CAD build for the part. Positions are in the model's coordinates, mm. A direction names the side the tool comes from. Coordinates: 2 decimals unless noted, no trailing zeros. Write each loop counter-clockwise with the first axis right and the second up, starting at its lowest first coordinate (ties: lowest second). Pieces come first, ordered by that corner, then holes. Notation, with made-up numbers: (-34.75, -34.5) -> (-11.75, -34.5) arc R31 cw to (-11.75, -0.5) -> close; hole circle Ø5 at (50.5, -31). An arc over 180 degrees is marked (long way). Answer as CSV lines item,"result".
Autodesk Inventor part; units mm, degrees
ref_plane "Work Plane1" through (0, 0, -3.5) normal (0, 0, 1) x (1, 0, 0)
ref_plane "YZ Plane" through (0, 0, 0) normal (1, 0, 0) x (0, 1, 0)
ref_plane "XZ Plane" through (0, 0, 0) normal (0, 1, 0) x (-1, 0, 0)
sketch "Sketch1" plane through (0, 0, 0) normal (0, 0, 1) x (1, 0, 0)
  line L0 (-8.12, 0) -> (8.12, 0)
  line L1 (0, -19.7) -> (0, 10.05)
  circle A0 centre (0, 0) radius 5.8
  line L2 (-5.8, -15.45) -> (5.8, -15.45)
  line L3 (5.8, -15.45) -> (5.8, 5.8)
  line L4 (5.8, 5.8) -> (-5.8, 5.8)
  line L5 (-5.8, 5.8) -> (-5.8, -15.45)
  line L6 (-5.8, -15.45) -> (5.8, 5.8) construction
  line L7 (5.8, -15.45) -> (-5.8, 5.8) construction
  circle A1 centre (0, -5.95) radius 3
  point P0 (0, -4.825)
  point P1 (0, -8.95)
  dimension "d4" = 6
  dimension "d0" = 21.25
  dimension "d1" = 11.6
  dimension "d5" = 6.5
extrude "Extrusion1" add sketch "Sketch1" against normal blind 20.2
extrude "Extrusion2" add sketch "Sketch1" along normal blind 3.35 contours A0 L1 L0 | L0 L1 A1 A0 | L1 A0 L0 | L0 A0 A1 L1 | A1 L1 A0 | A0 L1 A1 | A1 A0 L1 | A0 A1 L1
sketch "Sketch2" plane through (0, 0, 3.35) normal (0, 0, 1) x (1, 0, 0)
  arc A0 (2.8604, -5.0456) -> (-2.8604, -5.0456) centre (0, 0) ccw
  arc A1 (-2.8604, -5.0456) -> (2.8604, -5.0456) centre (0, -5.95) ccw
  circle A2 centre (0, -5.95) radius 1
  circle A3 centre (0, 0) radius 2.85
  circle A4 centre (0, 0) radius 1.9
  circle A5 centre (0, 0) radius 1.875
  circle A6 centre (0, 0) radius 0.675
  dimension "d9" = 5.7
  dimension "d10" = 2
  dimension "d11" = 3.8
  dimension "d14" = 3.75
  dimension "d17" = 1.35
extrude "Extrusion3" add sketch "Sketch2" along normal blind 0.6 contours A2 | A3
extrude "Extrusion4" add sketch "Sketch2" along normal blind 2.95 contours A5
ref_plane "Work Plane1" through (0, 0, -3.5) normal (0, 0, 1) x (1, 0, 0)
sketch "Sketch3" plane through (0, 0, -3.5) normal (0, 0, 1) x (1, 0, 0)
  line L0 (5.8, 5.8) -> (0, 5.8)
  line L1 (-5.8, 5.8) -> (5.8, 5.8)
  line L2 (0, 5.8) -> (-5.8, 5.8)
  line L3 (-5.8, -15.45) -> (5.8, -15.45)
  line L4 (5.8, -15.45) -> (-5.8, -15.45)
  line L5 (0, -19.7) -> (0, 10.05)
  line L6 (-5.8, 5.8) -> (-5.8, 0)
  line L7 (-5.8, -15.45) -> (-5.8, 5.8)
  line L8 (-5.8, 0) -> (-5.8, -15.45)
  line L9 (5.8, -15.45) -> (5.8, 0)
  line L10 (5.8, 5.8) -> (5.8, -15.45)
  line L11 (5.8, 0) -> (5.8, 5.8)
  line L12 (5.8, -4.825) -> (-5.8, -4.825)
  line L13 (-4.5, 5.8) -> (4.5, 5.8)
  line L14 (4.5, 5.8) -> (4, 10.05)
  line L15 (4, 10.05) -> (-4, 10.05)
  line L16 (-4, 10.05) -> (-4.5, 5.8)
  circle A0 centre (0, 7.875) radius 0.75
  line L17 (-4.5, -15.45) -> (4.5, -15.45)
  line L18 (4.5, -15.45) -> (4, -19.7)
  line L19 (4, -19.7) -> (-4, -19.7)
  line L20 (-4, -19.7) -> (-4.5, -15.45)
  circle A1 centre (0, -17.525) radius 0.75
  point P0 (0, 0)
  dimension "d19" = 1.5
  dimension "d20" = 9
  dimension "d21" = 8
  dimension "d22" = 4.25
  dimension "d23" = 25.4
extrude "Extrusion5" add sketch "Sketch3" against normal blind 0.9 contours L0 L5 A0 L15 L14 | L1 L16 L15 L5 A0 | L5 A1 L19 L20 L3 | L3 L18 L19 L5 A1
fillet "Fillet1" radius 1 4 edges at (4, -19.7, -3.95) (-4, -19.7, -3.95) (4, 10.05, -3.95) (-4, 10.05, -3.95)
chamfer "Chamfer1" distance 1.5 angle 45 1 edges at (0, 5.8, -20.2)
sketch "Sketch4" plane through (0, 0, -4.4) normal (0, 0, -1) x (-1, 0, 0)
  arc A0 (4.1039, 9.1668) -> (3.1108, 10.05) centre (3.1108, 9.05) ccw
  line L0 (3.1108, 10.05) -> (-3.1108, 10.05)
  arc A1 (-3.1108, 10.05) -> (-4.1039, 9.1668) centre (-3.1108, 9.05) ccw
  line L1 (-4.1039, 9.1668) -> (-4.5, 5.8)
  line L2 (4.5, 5.8) -> (-4.5, 5.8)
  line L3 (4.5, 5.8) -> (4.1039, 9.1668)
  circle A2 centre (0, 7.875) radius 0.75
  point P0 (0, 0)
extrude "BREAK_DA_TAB" [suppressed]
properties part number "empty"
Item 1: Saw through at B-B on x = -5. Give the cut face in (y, z), and give its area (3 significant figures).
Answer below:
outline,"(-15.45, -20.2) -> (4.3, -20.2) -> (5.8, -18.7) -> (5.8, 0) -> (2.94, 0) -> (2.94, 3.35) -> (-2.94, 3.35) -> (-2.94, 0) -> (-15.45, 0) -> close"
area,"448 mm2"
Item 2: Flat gauge pins, fed straight in: pin 1 (4.5 mm diameter, centred on x = 0.5, y = 8, fed in from -Z); pin 2 (2 mm diameter, centred on x = -2, y = -18, fed in from +Z); pin 3 (3.5 mm diameter, centred on x = 2.5, y = -11, fed in from +Z); pin 4 (0.9 mm diameter, centred on x = 0, y = 7.875, fed in from -Z). Where does each tip first touch, or does it go through?
Answer below:
pin 1,"stops at z = -18.75"
pin 2,"stops at z = -3.5"
pin 3,"stops at z = 0"
pin 4,"passes through"
Item 3: Saw through at D-D on y = -9.5. Give the cut face in (x, z).
Answer below:
outline,"(-5.8, -20.2) -> (5.8, -20.2) -> (5.8, 0) -> (-5.8, 0) -> close"
Item 4: Saw through at A-A on y = -5.95. Give the cut face in (x, z).
Answer below:
outline,"(-5.8, -20.2) -> (5.8, -20.2) -> (5.8, 0) -> (3, 0) -> (3, 3.35) -> (1, 3.35) -> (1, 3.95) -> (-1, 3.95) -> (-1, 3.35) -> (-3, 3.35) -> (-3, 0) -> (-5.8, 0) -> close"
Item 5: Wall check: line 1 (Y direction, x = 0, z = -4) (3 decimals); line 2 (Y direction, x = 0, z = 4.95) (3 decimals); line 3 (Y direction, x = 2.5, z = -1.25). Give the ranges that are in metal, low to high. Write a range as from..to.
Answer below:
line 1,"y = -19.7..-18.275, -16.775..7.125, 8.625..10.05"
line 2,"y = -1.875..-0.675, 0.675..1.875"
line 3,"y = -15.45..5.8"
Item 6: Saw through at C-C on z = -12.5. Give the cut face in (x, y).
Answer below:
outline,"(-5.8, -15.45) -> (5.8, -15.45) -> (5.8, 5.8) -> (-5.8, 5.8) -> close"
Item 7: Two-plate mould, pull along X, no slides. Class faces 1 (the cylindrical face through (-0.1, -16.78, -3.94)), 2 (the cylindrical face through (-0.217, -4.974, 3.646)), 3 (the flat face through (-4.3, 7.5, -3.9)): pulls with the +X half, pulls with the -X half, needs draft (parallel to the pull), parting line crosses it, or undercut.
Answer below:
face 1,"undercut"
face 2,"parting line crosses it"
face 3,"pulls with the -X half"
Item 8: 3-axis set-ups, long thin cutter, end or side, ignore diameter. For faces 4 (the flat face through (0, -5, -20.2)), 5 (the cylindrical face through (-2.262, 1.734, 3.646)): which of +Z, -Z, +X, -X, +Y, -Y reach the whole face in a straight line?
Answer below:
face 4,"-Z, +X, -X, +Y, -Y"
face 5,"+Z"
